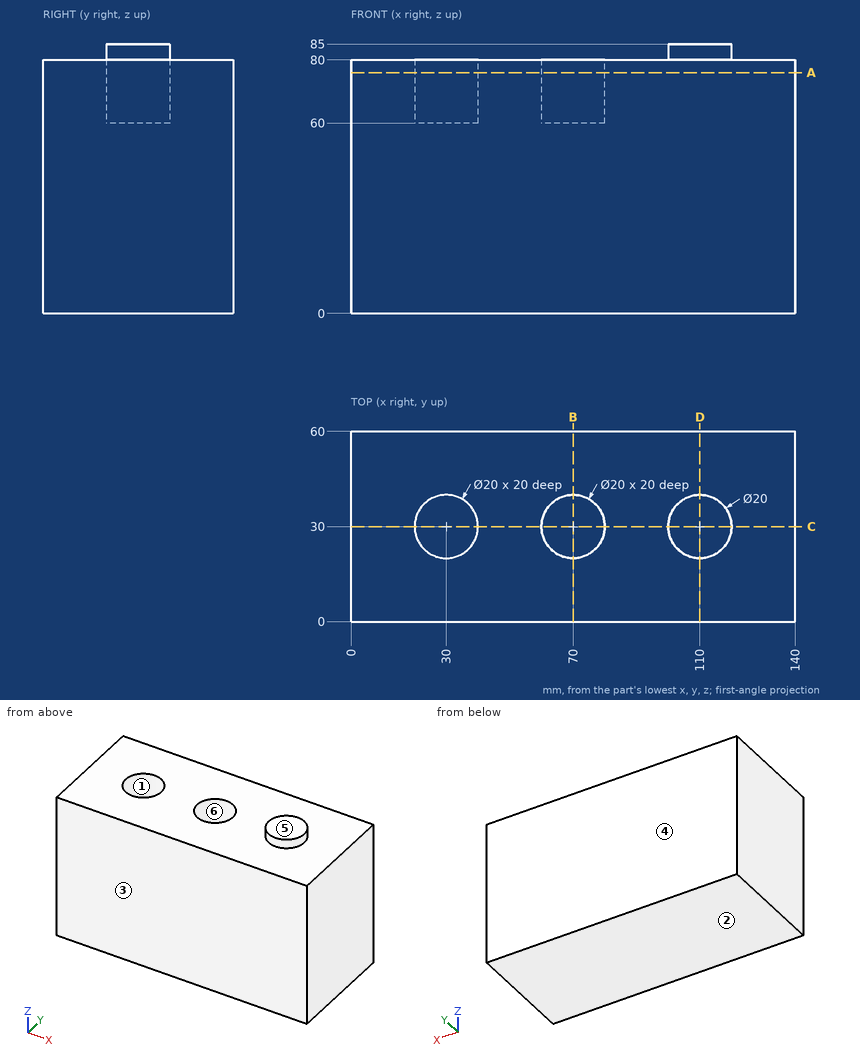
Job drawing, mm, ordinate dimensions from the low corner. One solid piece. A direction names the side the tool comes from. Round coordinates to 2 decimals unless told otherwise and drop trailing zeros. Loops run counter-clockwise (first coordinate to the right, second up) from the corner with the lowest first, then second, coordinate; pieces in that order, holes last. Notation, with made-up numbers: (50.5, -24.75) -> (70.5, -24.75) arc R19 cw to (70.5, -0.75) -> close; hole circle Ø11 at (21.25, 34). An arc over 180 degrees is marked (long way). Use a Markdown table: item, result.
1) Cut at B-B, the plane x = 70. List the corners of the cut face in (y, z).
The answers:
| item | result |
|---|---|
| outline | (0, 0) -> (60, 0) -> (60, 80) -> (40, 80) -> (40, 60) -> (20, 60) -> (20, 80) -> (0, 80) -> close |
2) Cut at C-C, the plane y = 30. List the corners of the cut face in (x, z).
The answers:
| item | result |
|---|---|
| outline | (0, 0) -> (140, 0) -> (140, 80) -> (120, 80) -> (120, 85) -> (100, 85) -> (100, 80) -> (80, 80) -> (80, 60) -> (60, 60) -> (60, 80) -> (40, 80) -> (40, 60) -> (20, 60) -> (20, 80) -> (0, 80) -> close |
3) Drop flat-ended pins along their axis: pin 1 Ø2 at (x, y) = (114, 13) entering from +Z; pin 2 Ø12 at (x, y) = (30, 30) entering from +Z. Give the stop position or say it passes through.
The answers:
| item | result |
|---|---|
| pin 1 | stops at z = 80 |
| pin 2 | stops at z = 60 |
4) Cut at D-D, the plane x = 110. List the corners of the cut face in (y, z), and give its area (3 significant figures).
The answers:
| item | result |
|---|---|
| outline | (0, 0) -> (60, 0) -> (60, 80) -> (40, 80) -> (40, 85) -> (20, 85) -> (20, 80) -> (0, 80) -> close |
| area | 4,900 mm2 |
5) Cut at A-A, the plane z = 76. List the corners of the cut face in (x, y).
The answers:
| item | result |
|---|---|
| outline | (0, 0) -> (140, 0) -> (140, 60) -> (0, 60) -> close; hole circle Ø20 at (30, 30); hole circle Ø20 at (70, 30) |
6) Pull direction Y, two halves, no side cores. Call the marked faces 3, 4, 5 and 6: pulls with the +Y half, pulls with the -Y half, needs draft (parallel to the pull), parting line crosses it, or undercut.
The answers:
| item | result |
|---|---|
| face 3 | pulls with the -Y half |
| face 4 | pulls with the +Y half |
| face 5 | needs draft |
| face 6 | undercut |
7) Probe line 1 (Y direction, x = 30, z = 74); line 2 (Z direction, x = 90, y = 31); line 3 (X direction, y = 34, z = 66). List the from-to ranges inside material, lowest first. Write a range as [from, to].
The answers:
| item | result |
|---|---|
| line 1 | y = [0, 20], [40, 60] |
| line 2 | z = [0, 80] |
| line 3 | x = [0, 20.83], [39.17, 60.83], [79.17, 140] |
8) Tool access for the marked faces 1 and 2: list every direction of +Z, -Z, +X, -X, +Y, -Y with a clear straight run to the whole face (end or side of a thin tool).
The answers:
| item | result |
|---|---|
| face 1 | +Z |
| face 2 | -Z, +X, -X, +Y, -Y |
